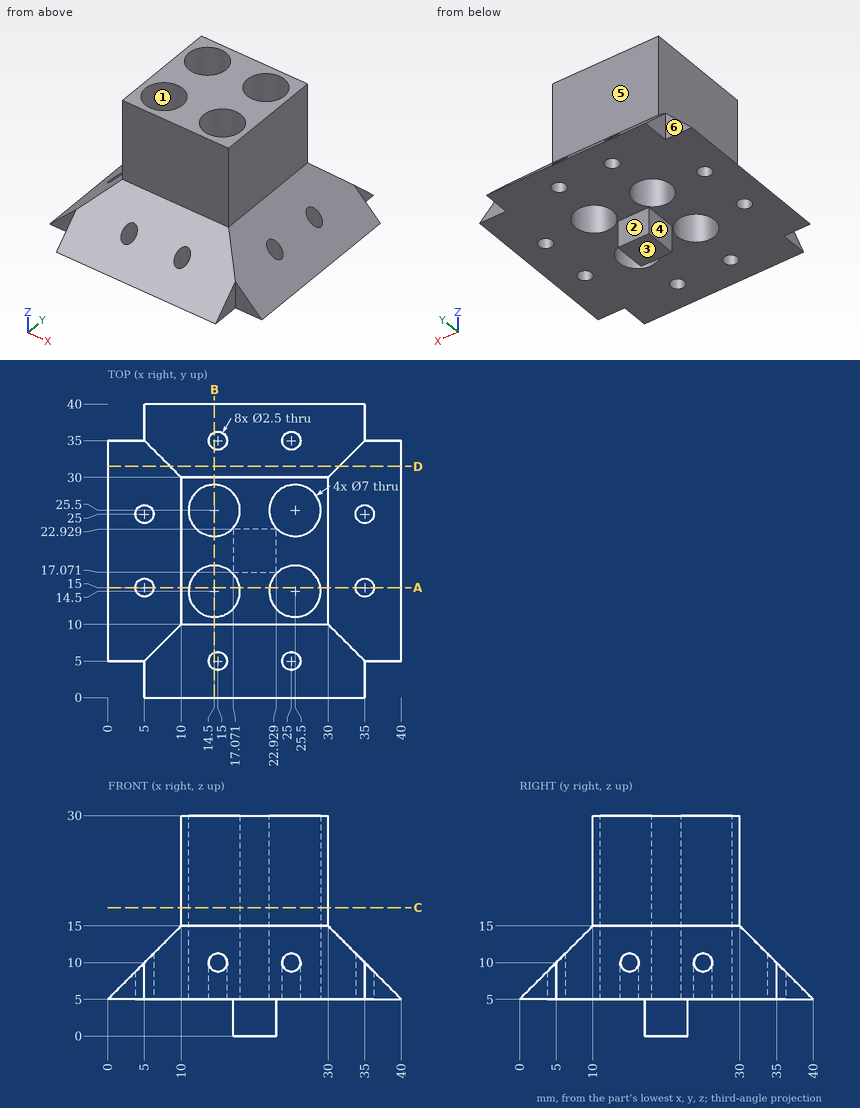
Verification items for this drawing (mm, ordinates from the low corner). A direction names the side the tool comes from. Coordinates: 2 decimals unless noted, no trailing zeros. Loops run counter-clockwise (first coordinate to the right, second up) from the corner with the lowest first, then second, coordinate; pieces in that order, holes last. Notation, with made-up numbers: (68, -16.5) -> (83, -16.5) arc R19 cw to (83, 3.5) -> close; hole circle Ø7 at (-12.75, 56). An arc over 180 degrees is marked (long way). Answer in a Markdown table with one row per item. Add a question column.
1. Access from +Z, -Z, +X, -X, +Y, -Y to the whole of each face (thin tool, end or side, straight path). Record for the marked faces 4, 5 and 6.
2. Section check C-C, the plane z = 17.5. Enter the section's corners in (x, y), then the cut area to 3 significant figures.
3. Section check D-D, the plane y = 31.5. Enter the section's corners in (x, z).
4. Section check A-A, the plane y = 15. Enter the section's corners in (x, z), then the cut area to 3 significant figures.
5. Depth check by flat-ended pin: P1, Ø2.5, axis at x = 19.5, z = 2, coming from the -Y side; P2, Ø4, axis at x = 14.5, y = 14.5, coming from the +Z side; P3, Ø2.5, axis at x = 36.5, z = 8.5, coming from the +Y side; P4, Ø2.5, axis at x = 20, z = 3.5, coming from the +Y side. Enter the tip coordinate at first touch or a pass-through.
6. Section check B-B, the plane x = 14.5. Enter the section's corners in (y, z).
7. Material ranges on probe 1 along X at (y, z) = (25, 9.5); probe 2 along Y at (x, z) = (6, 8); probe 3 along X at (y, z) = (24, 12.5), recorded low to high. Write a range as [from, to].
8. Draft check along Y on the marked faces 1, 2 and 3. Enter one of: +Y half, -Y half, draft (parallel to the pull), parting line (faces both ways), or undercut.
Derived:
| question | item | result |
|---|---|---|
| 1 | face 4 | -Z, -X, +Y, -Y |
| 1 | face 5 | +Z, +X, -X, +Y |
| 1 | face 6 | +Z, -Z, -X, +Y |
| 2 | outline | (10, 10) -> (30, 10) -> (30, 30) -> (10, 30) -> close; hole circle Ø7 at (14.5, 14.5); hole circle Ø7 at (14.5, 25.5); hole circle Ø7 at (25.5, 14.5); hole circle Ø7 at (25.5, 25.5) |
| 2 | area | 246 mm² |
| 3 | outline | (0, 5) -> (40, 5) -> (31.5, 13.5) -> (8.5, 13.5) -> close |
| 4 | outline | (0, 5) -> (3.75, 5) -> (3.75, 8.75) -> close; (6.25, 5) -> (11.04, 5) -> (11.04, 30) -> (10, 30) -> (10, 15) -> (6.25, 11.25) -> close; (17.96, 5) -> (22.04, 5) -> (22.04, 30) -> (17.96, 30) -> close; (28.96, 5) -> (33.75, 5) -> (33.75, 11.25) -> (30, 15) -> (30, 30) -> (28.96, 30) -> close; (36.25, 5) -> (40, 5) -> (36.25, 8.75) -> close |
| 4 | area | 229 mm² |
| 5 | P1 | stops at y = 17.07 |
| 5 | P2 | passes through |
| 5 | P3 | stops at y = 35 |
| 5 | P4 | stops at y = 22.93 |
| 6 | outline | (0, 5) -> (3.85, 5) -> (3.85, 8.85) -> close; (6.15, 5) -> (11, 5) -> (11, 30) -> (10, 30) -> (10, 15) -> (6.15, 11.15) -> close; (18, 5) -> (22, 5) -> (22, 30) -> (18, 30) -> close; (29, 5) -> (33.85, 5) -> (33.85, 11.15) -> (30, 15) -> (30, 30) -> (29, 30) -> close; (36.15, 5) -> (40, 5) -> (36.15, 8.85) -> close |
| 7 | probe 1 | x = [6.25, 11.04], [17.96, 22.04], [28.96, 33.75] |
| 7 | probe 2 | y = [3, 14.25], [15.75, 24.25], [25.75, 37] |
| 7 | probe 3 | x = [7.5, 11.34], [17.66, 22.34], [28.66, 32.5] |
| 8 | face 1 | undercut |
| 8 | face 2 | +Y half |
| 8 | face 3 | draft |
